```python
from build123d import *


with BuildPart() as f1:
    # F0 (on Front) → F1 (revolve)
    with BuildSketch(Plane.XZ):
        Polygon((-10.5, 0), (-1.5, 0), (-1.5, 3.5), (-12, 3.5), (-12, 2), align=None)
        Polygon((-1.5, -3.5), (-1.5, 0), (-10.5, 0), (-12, -2), (-12, -3.5), align=None)
    revolve(axis=Axis((0, 0, 1), (0, 0, 1)))


solid = f1.part
```
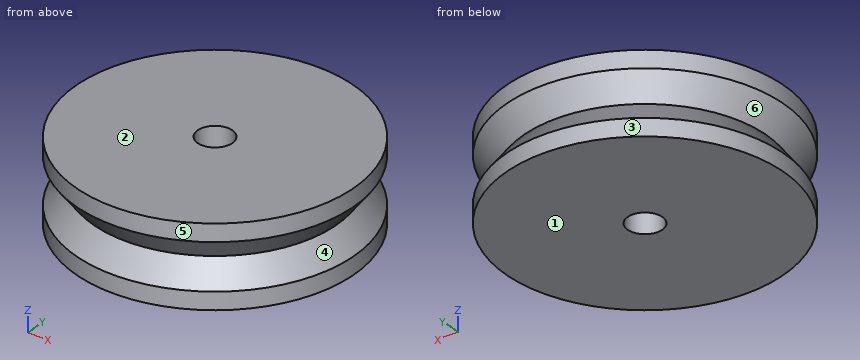
Part model, mm, in its own coordinate system. Face numbers are marked on the shaded views. A direction names the side the tool comes from. Coordinates: 2 decimals unless noted, no trailing zeros. Order: outer loops, then holes, each group sorted by start corner. A loop starts at its lowest first (then second) coordinate and runs counter-clockwise, first axis right, second up. Notation, with made-up numbers: (73.5, 22.25) -> (78.5, 22.25) arc R28 cw to (78.5, 54.25) -> close; hole circle Ø7 at (12.5, 28). An arc over 180 degrees is marked (long way). Put each result on its own line as item: value. Start each with the question number.
(1) Mould opens along Z. For the marked faces 1, 2, 3 and 4 say: pulls with the +Z half, pulls with the -Z half, needs draft (parallel to the pull), parting line crosses it, or undercut.
(2) Probe line 1 along Y through (x, z) = (0, -2); line 2 along Z through (x, y) = (9.75, -4.75). List the from-to ranges inside material, lowest first. Write a range as [from, to].
(3) Which spindle directions (+Z, -Z, +X, -X, +Y, -Y) get a long thin tool onto all of the face, cutting with end or side? Do the marked faces 5 and 6. Say none if no direction does.
(4) Band-saw the part on A-A (x = 0). Give the cut face in (y, z).
(5) Pin check, flat tips, straight feed: pin 1 Ø2 at (y, z) = (3, 1.5) entering from -X; pin 2 Ø2.5 at (x, y) = (0, 0) entering from -Z. Stop position of each tip, or through.
(6) Band-saw the part on C-C (z = 3). Give the cut face in (x, y), then the cut area to 3 significant figures.
(7) Band-saw the part on D-D (z = 0.75). Give the cut face in (x, y) (1 decimal), then the cut area to 3 significant figures.
Determined:
1. face 1: pulls with the -Z half
1. face 2: pulls with the +Z half
1. face 3: needs draft
1. face 4: undercut
2. line 1: y = [-12, -1.5], [1.5, 12]
2. line 2: z = [-3.5, -0.46], [0.46, 3.5]
3. face 5: +Z, -Z
3. face 6: none
4. outline: (-12, -3.5) -> (-1.5, -3.5) -> (-1.5, 3.5) -> (-12, 3.5) -> (-12, 2) -> (-10.5, 0) -> (-12, -2) -> close; (1.5, -3.5) -> (12, -3.5) -> (12, -2) -> (10.5, 0) -> (12, 2) -> (12, 3.5) -> (1.5, 3.5) -> close
5. pin 1: stops at x = -11.81
5. pin 2: passes through
6. outline: circle Ø24 at (0, 0); hole circle Ø3 at (0, 0)
6. area: 445 mm²
7. outline: circle Ø22.1 at (0, 0); hole circle Ø3 at (0, 0)
7. area: 377 mm²
